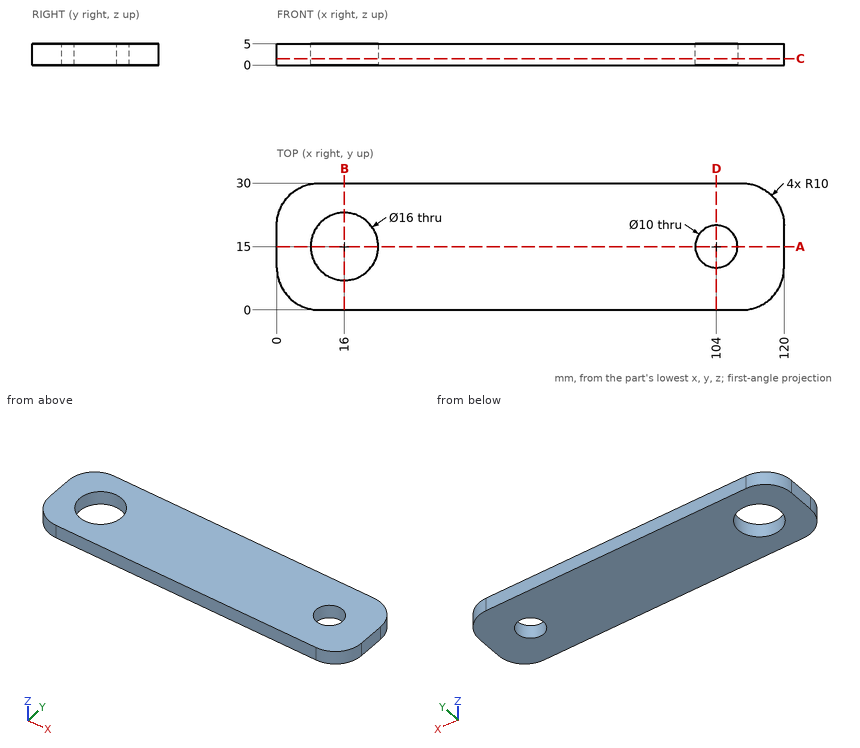
Part print with two shaded views. Sizes in mm from the minimum x, y, z corner. Round coordinates to 2 decimals unless told otherwise and drop trailing zeros. Order: outer loops, then holes, each group sorted by start corner. A loop starts at its lowest first (then second) coordinate and runs counter-clockwise, first axis right, second up. Notation, with made-up numbers: M -37,-27 L -12,-27 A19 ccw -12,-14 Z; hole C 82,-15 d5. An arc over 180 degrees is marked long. Put each result on its own line as item: value. Start each with the question number.
1. Slice it at B-B on x = 16. List the corners of the cut face in (y, z).
2. Slice it at C-C on z = 1.55. List the corners of the cut face in (x, y).
3. Slice it at D-D on x = 104. List the corners of the cut face in (y, z), then the cut area to 3 significant figures.
4. Slice it at A-A on y = 15. List the corners of the cut face in (x, z).
5. Drop flat-ended pins along their axis: pin 1 (3 mm diameter, centred on y = 15.5, z = 2.5, fed in from -X); pin 2 (2 mm diameter, centred on y = 25.5, z = 2, fed in from -X). Give the stop position or say it passes through.
6. Drill centre lines: probe 1 along Y at (x, z) = (16, 2.75); probe 2 along X at (y, z) = (14, 4); probe 3 along X at (y, z) = (12.5, 2.65). Where is each one in solid material? Low to high. Write a range as [from, to].
Findings:
1. outline: M 0,0 L 7,0 L 7,5 L 0,5 Z; M 23,0 L 30,0 L 30,5 L 23,5 Z
2. outline: M 0,10 A10 ccw 10,0 L 110,0 A10 ccw 120,10 L 120,20 A10 ccw 110,30 L 10,30 A10 ccw 0,20 Z; hole C 16,15 d16; hole C 104,15 d10
3. outline: M 0,0 L 10,0 L 10,5 L 0,5 Z; M 20,0 L 30,0 L 30,5 L 20,5 Z
3. area: 100 mm2
4. outline: M 0,0 L 8,0 L 8,5 L 0,5 Z; M 24,0 L 99,0 L 99,5 L 24,5 Z; M 109,0 L 120,0 L 120,5 L 109,5 Z
5. pin 1: x = 0
5. pin 2: x = 1.07
6. probe 1: [0, 7], [23, 30]
6. probe 2: [0, 8.06], [23.94, 99.1], [108.9, 120]
6. probe 3: [0, 8.4], [23.6, 99.67], [108.33, 120]
